from build123d import *

# Parameters (mm, degrees)
SKETCH1_W               = 383.54
SKETCH1_H               = 228.6
BOSS_EXTRUDE1_DEPTH     = 5.08
CUT_EXTRUDE4_DEPTH      = 2.54
CUT_EXTRUDE4_DEPTH_BACK = 2.032
SKETCH3_W               = 7.551410014
SKETCH3_H               = 7.624040678
SKETCH3_W_2             = 8.426229182
SKETCH3_W_3             = 7.372950534
SKETCH3_H_2             = 8.377243284
SKETCH3_H_3             = 7.836309586
SKETCH3_H_4             = 23.885974754
SKETCH3_W_4             = 7.738672286
SKETCH3_W_5             = 8.057581655
SKETCH3_W_6             = 7.668237515
SKETCH3_H_5             = 12.138714326
SKETCH3_H_6             = 7.824594082
SKETCH3_H_7             = 20.136219216
SKETCH3_W_7             = 15.20808594
SKETCH3_H_8             = 7.579699467
SKETCH3_W_8             = 7.446662222
SKETCH3_W_9             = 13.868168861
SKETCH3_H_9             = 7.623435987
SKETCH3_H_10            = 12.134909421
SKETCH3_H_11            = 7.62
SKETCH3_W_10            = 7.699091451
SKETCH3_W_11            = 7.508994489
SKETCH3_H_12            = 12.721182216
SKETCH3_H_13            = 7.933797838
SKETCH3_W_12            = 15.145753673
SKETCH3_W_13            = 7.502078631
SKETCH3_W_14            = 7.480081761
SKETCH3_H_14            = 7.922088466
SKETCH3_H_15            = 7.672421885
SKETCH3_H_16            = 12.219933912
SKETCH3_H_17            = 7.494674976
SKETCH3_W_15            = 10.718331987
SKETCH3_H_18            = 7.528655491
SKETCH3_H_19            = 7.933797839
SKETCH3_W_16            = 3.019240536
SKETCH3_W_17            = 4.489753953
SKETCH3_H_20            = 12.727502234
SKETCH4_W               = 383.54
SKETCH4_H               = 25.463727846
SKETCH4_H_2             = 25.336272154
CUT_EXTRUDE5_DEPTH      = 6.35
SKETCH7_R               = 3.302
SKETCH7_R_2             = 11.43
CUT_EXTRUDE6_DEPTH      = 203.2
SKETCH8_W               = 15.24
SKETCH8_H               = 5.08
BOSS_EXTRUDE2_DEPTH     = 20.32
SKETCH11_R              = 1.5
CUT_EXTRUDE7_DEPTH      = 381


with BuildPart() as part:
    # Sketch1 → Boss-Extrude1 (new body)
    with BuildSketch(Plane.XY):
        Rectangle(SKETCH1_W, SKETCH1_H)
    extrude(amount=BOSS_EXTRUDE1_DEPTH)

    # Sketch3 → Cut-Extrude4 (cut, two sides: drawn at the far end of the back side and taken through both)
    with BuildSketch(Plane.XY.offset(5.08).offset(-CUT_EXTRUDE4_DEPTH_BACK)):
        with Locations((-72.346363981, 20.182774132)):
            Rectangle(SKETCH3_W, SKETCH3_H)
        with Locations((-64.357544383, 20.182774132)):
            Rectangle(SKETCH3_W_2, SKETCH3_H)
        with Locations((-56.457954525, 20.182774132)):
            Rectangle(SKETCH3_W_3, SKETCH3_H)
        with Locations((-56.457954525, 12.182132151)):
            Rectangle(SKETCH3_W_3, SKETCH3_H_2)
        with Locations((-72.346363981, 4.075355716)):
            Rectangle(SKETCH3_W, SKETCH3_H_3)
        with Locations((-72.346363981, -11.785786454)):
            Rectangle(SKETCH3_W, SKETCH3_H_4)
        with Locations((-72.346363981, 12.182132151)):
            Rectangle(SKETCH3_W, SKETCH3_H_2)
        with Locations((-64.357544383, 12.182132151)):
            Rectangle(SKETCH3_W_2, SKETCH3_H_2)
        Polygon((-68.570658974, 7.993510509), (-68.570658974, 0.157200923), (-60.950658974, 0.157200923), (-52.771479258, 0.157200923), (-52.771479258, 7.993510509), (-60.144429792, 7.993510509), align=None)
        Polygon((-68.570658974, 0.157200923), (-59.968883351, -23.728773831), (-52.348883351, -23.728773831), (-60.950658974, 0.157200923), align=None)
        with Locations((-44.220529343, 20.182774132)):
            Rectangle(SKETCH3_W_4, SKETCH3_H)
        with Locations((-36.322402373, 20.182774132)):
            Rectangle(SKETCH3_W_5, SKETCH3_H)
        with Locations((-28.459492788, 20.182774132)):
            Rectangle(SKETCH3_W_6, SKETCH3_H)
        with Locations((-28.459492788, 10.30139663)):
            Rectangle(SKETCH3_W_6, SKETCH3_H_5)
        with Locations((-36.322402373, 10.30139663)):
            Rectangle(SKETCH3_W_5, SKETCH3_H_5)
        with Locations((-44.220529343, 10.30139663)):
            Rectangle(SKETCH3_W_4, SKETCH3_H_5)
        with Locations((-44.220529343, 0.319742426)):
            Rectangle(SKETCH3_W_4, SKETCH3_H_6)
        with Locations((-36.322402373, 0.319742426)):
            Rectangle(SKETCH3_W_5, SKETCH3_H_6)
        Polygon((-24.62537403, 0.157200923), (-24.62537403, 4.232039467), (-32.293611545, 4.232039467), (-32.293611545, -3.592554615), (-24.62537403, -3.592554615), align=None)
        with Locations((-44.220529343, -13.660664223)):
            Rectangle(SKETCH3_W_4, SKETCH3_H_7)
        with Locations((-28.459492788, -13.660664223)):
            Rectangle(SKETCH3_W_6, SKETCH3_H_7)
        Polygon((-12.735071294, 23.994794471), (-20.70205372, 23.994794471), (-20.70205372, -23.994794471), (-12.735071294, -23.994794471), (-12.735071294, 10.313389338), align=None)
        Polygon((-8.004675478, 16.370753793), (-12.735071294, 23.994794471), (-12.735071294, 10.313389338), (-8.004675478, 2.426315091), (-3.274279663, 10.208504268), (-3.274279663, 23.994794471), align=None)
        Polygon((4.360745163, 23.994794471), (-3.274279663, 23.994794471), (-3.274279663, 10.208504268), (-3.274279663, -23.994794471), (4.360745163, -23.994794471), align=None)
        with Locations((22.317437477, 20.204944737)):
            Rectangle(SKETCH3_W_7, SKETCH3_H_8)
        with Locations((10.990063396, 20.204944737)):
            Rectangle(SKETCH3_W_8, SKETCH3_H_8)
        with Locations((48.563017268, 20.072456114)):
            Rectangle(SKETCH3_W_9, SKETCH3_H_9)
        with Locations((10.990063396, 10.347640294)):
            Rectangle(SKETCH3_W_8, SKETCH3_H_10)
        with Locations((10.990063396, 0.470185583)):
            Rectangle(SKETCH3_W_8, SKETCH3_H_11)
        with Locations((18.562940233, 0.470185583)):
            Rectangle(SKETCH3_W_10, SKETCH3_H_11)
        with Locations((26.166983202, 0.470185583)):
            Rectangle(SKETCH3_W_11, SKETCH3_H_11)
        with Locations((26.166983202, -9.700405525)):
            Rectangle(SKETCH3_W_11, SKETCH3_H_12)
        with Locations((26.166983202, -20.027895552)):
            Rectangle(SKETCH3_W_11, SKETCH3_H_13)
        with Locations((14.839609122, -20.027895552)):
            Rectangle(SKETCH3_W_12, SKETCH3_H_13)
        with Locations((37.877893521, 20.072456114)):
            Rectangle(SKETCH3_W_13, SKETCH3_H_9)
        Polygon((41.628932837, 16.26073812), (34.126854206, 16.26073812), (34.126854206, -16.215353517), (41.628932837, -16.215353517), (41.628932837, -4.115401118), (34.148851076, -4.115401118), (34.148851076, 3.806687348), (41.628932837, 3.806687348), align=None)
        with Locations((37.888891957, -0.154356885)):
            Rectangle(SKETCH3_W_14, SKETCH3_H_14)
        with Locations((45.368973717, -0.154356885)):
            Rectangle(SKETCH3_W_14, SKETCH3_H_14)
        with Locations((37.877893521, -20.051564459)):
            Rectangle(SKETCH3_W_13, SKETCH3_H_15)
        with Locations((48.563017268, -20.051564459)):
            Rectangle(SKETCH3_W_9, SKETCH3_H_15)
        with Locations((61.68040589, 10.390152539)):
            Rectangle(SKETCH3_W_8, SKETCH3_H_16)
        with Locations((61.68040589, 20.247456983)):
            Rectangle(SKETCH3_W_8, SKETCH3_H_17)
        with Locations((70.762902995, 20.247456983)):
            Rectangle(SKETCH3_W_15, SKETCH3_H_17)
        Polygon((65.403737001, 24.079818962), (65.403737001, 23.994794471), (76.122068988, 23.994794471), (76.122068988, 16.500119495), (80.611822941, 16.500119495), (80.611822941, 24.079818962), align=None)
        with Locations((61.68040589, 0.515857838)):
            Rectangle(SKETCH3_W_8, SKETCH3_H_18)
        with Locations((65.529951616, -19.942871061)):
            Rectangle(SKETCH3_W_12, SKETCH3_H_19)
        with Locations((69.253282727, 0.515857838)):
            Rectangle(SKETCH3_W_10, SKETCH3_H_18)
        with Locations((74.61244872, 0.515857838)):
            Rectangle(SKETCH3_W_16, SKETCH3_H_18)
        with Locations((78.366945965, 0.515857838)):
            Rectangle(SKETCH3_W_17, SKETCH3_H_18)
        with Locations((78.366945965, -9.612221025)):
            Rectangle(SKETCH3_W_17, SKETCH3_H_20)
        with Locations((74.61244872, -9.612221025)):
            Rectangle(SKETCH3_W_16, SKETCH3_H_20)
        with Locations((74.61244872, -19.942871061)):
            Rectangle(SKETCH3_W_16, SKETCH3_H_19)
        with Locations((78.366945965, -19.942871061)):
            Rectangle(SKETCH3_W_17, SKETCH3_H_19)
    extrude(amount=CUT_EXTRUDE4_DEPTH + CUT_EXTRUDE4_DEPTH_BACK, mode=Mode.SUBTRACT)

    # Sketch4 → Cut-Extrude5 (cut)
    with BuildSketch(Plane.XY.offset(5.08)):
        with Locations((0, 101.568136077)):
            Rectangle(SKETCH4_W, SKETCH4_H)
        with Locations((0, -101.631863923)):
            Rectangle(SKETCH4_W, SKETCH4_H_2)
    extrude(amount=-CUT_EXTRUDE5_DEPTH, mode=Mode.SUBTRACT)

    # Sketch7 → Cut-Extrude6 (cut)
    with BuildSketch(Plane.XY.offset(5.08)):
        with Locations((93.506776136, -0.23396958)):
            Circle(SKETCH7_R)
        with Locations((111.540776136, -0.23396958)):
            Circle(SKETCH7_R_2)
        with Locations((129.604477858, -0.23396958)):
            Circle(SKETCH7_R)
    extrude(amount=-CUT_EXTRUDE6_DEPTH, mode=Mode.SUBTRACT)

    # Sketch8 → Boss-Extrude2 (add)
    with BuildSketch(Plane.XY.offset(5.08)):
        Polygon((16.51, 93.916272154), (-196.85, 93.916272154), (-196.85, -94.043727846), (16.51, -94.043727846), (16.51, -88.963727846), (-191.77, -88.963727846), (-191.77, 88.836272154), (16.51, 88.836272154), align=None)
        with Locations((189.23, 91.376272154)):
            Rectangle(SKETCH8_W, SKETCH8_H)
        Polygon((196.85, 88.835766484), (191.77, 88.835766484), (191.77, -88.963727846), (181.61, -88.963727846), (181.61, -94.043727846), (196.85, -94.043727846), align=None)
    extrude(amount=-BOSS_EXTRUDE2_DEPTH)

    # Sketch11 → Cut-Extrude7 (cut)
    with BuildSketch(Plane.XZ.offset(94.043727846)):
        with Locations((-158.75, -10.16)):
            Circle(SKETCH11_R)
        with Locations((-95.25, -10.16)):
            Circle(SKETCH11_R)
        with Locations(Location((184.15, -10.16, 0), (0, 0, 270))):
            Circle(SKETCH11_R)
        with Locations((-31.75, -10.16)):
            Circle(SKETCH11_R)
    extrude(amount=-CUT_EXTRUDE7_DEPTH, mode=Mode.SUBTRACT)


solid = part.part
Work out the finished part from the listing and answer in its coordinate system (mm). A direction names the side the tool comes from. Give positions to 0.01 mm unless a question says otherwise; leave off trailing zeros. Loops run counter-clockwise (first coordinate to the right, second up) from the corner with the lowest first, then second, coordinate; pieces in that order, holes last. Notation, with made-up numbers: (21, 73.25) -> (69, 73.25) arc R20 ccw to (69, 110.25) -> close; hole circle Ø4 at (14, 5). An arc over 180 degrees is marked (long way). Use a Markdown table: item, result. Add a question column.
1) For a pull along X with two mould halves and no side action, classify faces 6 (the flat face through (-3, 43, 5.08)), 7 (the flat face through (-8, 6, 3.048)), 8 (the flat face through (196.85, -4, -5)), 9 (the flat face through (-196.85, 1, -5)) as +X half, -X half, draft (parallel to the pull), parting line (faces both ways), or undercut.
2) The part is cut by section B-B, the plane x = 113.5. Determine the outline of the cut face in (y, z), plus the area to 3 significant figures.
3) Which of the six approach directions +Z, -Z, +X, -X, +Y, -Y give full straight-line access (tool end or side, diameter ignored) to faces 1 (the flat face through (-56.59, -11.95, 4.05)), 2 (the flat face through (187, -88.964, -8)), 3 (the flat face through (189, 88.836, -7)), 4 (the cylindrical face through (90.208, -0.089, 2.576)), 5 (the flat face through (-193, 0, -15.24))?
4) The part is cut by section C-C, the plane x = 155.5. Determine the outline of the cut face in (y, z), plus the area to 3 significant figures.
5) The part is cut by section A-A, the plane y = 29.5. Determine the outline of the cut face in (x, z).
6) Consider line 1 along Y through (x, z) = (-30, -7); line 2 along Z through (x, y) = (-31.75, -92.9); line 3 along X through (y, z) = (-74, -13.75). Determine where each line is inside the solid, lowest interval first.
7) This flat-tipped pin is pushed along its axis until it touches: P1, Ø3, axis at x = 48.5, y = -6, coming from the -Z side. Where does it stop, or does it pass through?
Reported:
| question | item | result |
|---|---|---|
| 1 | face 6 | draft |
| 1 | face 7 | undercut |
| 1 | face 8 | +X half |
| 1 | face 9 | -X half |
| 2 | outline | (-88.96, 0) -> (-11.49, 0) -> (-11.49, 5.08) -> (-88.96, 5.08) -> close; (11.03, 0) -> (88.84, 0) -> (88.84, 5.08) -> (11.03, 5.08) -> close |
| 2 | area | 789 mm^2 |
| 3 | face 1 | +Z |
| 3 | face 2 | -Z |
| 3 | face 3 | none |
| 3 | face 4 | +Z, -Z |
| 3 | face 5 | -Z, +X, -X, +Y, -Y |
| 4 | outline | (-88.96, 0) -> (88.84, 0) -> (88.84, 5.08) -> (-88.96, 5.08) -> close |
| 4 | area | 903 mm^2 |
| 5 | outline | (-196.85, -15.24) -> (-191.77, -15.24) -> (-191.77, 0) -> (191.77, 0) -> (191.77, -15.24) -> (196.85, -15.24) -> (196.85, 5.08) -> (-196.85, 5.08) -> close |
| 6 | line 1 | y = -94.04 to -88.96, 88.84 to 93.92 |
| 6 | line 2 | z = -15.24 to -11.66, -8.66 to 5.08 |
| 6 | line 3 | x = -196.85 to -191.77, 191.77 to 196.85 |
| 7 | P1 | stops at z = 0 |
